Can you work these out from the model? Positions are in its coordinate system, mm. Give positions to 0.01 mm unless a question says otherwise; leave off trailing zeros. Order: outer loops, then holes, each group sorted by start corner. A loop starts at its lowest first (then second) coordinate and runs counter-clockwise, first axis right, second up. Notation, with made-up numbers: (77.25, 72) - (86.25, 72) arc R26 ccw to (86.25, 110) - close; hole circle Ø4 at (35.25, 82). An arc over 180 degrees is marked (long way). Write each question's results on one line, items separated by ' | '. Start each with the question number.
Autodesk Inventor part; units mm, degrees
ref_plane "YZ Plane" through (0, 0, 0) normal (1, 0, 0) x (0, 1, 0)
ref_plane "XZ Plane" through (0, 0, 0) normal (0, 1, 0) x (-1, 0, 0)
ref_plane "XY Plane" through (0, 0, 0) normal (0, 0, 1) x (1, 0, 0)
sketch "Skizze_1" plane through (0, 0, 0) normal (0, 0, 1) x (1, 0, 0)
  line L0 (-17.5, 0) -> (-17.5, -1)
  line L1 (-17.5, -1) -> (-13.5, -1)
  line L2 (-13.5, -1) -> (-13.5, -7.5)
  line L3 (-13.5, -7.5) -> (13.5, -7.5)
  line L4 (13.5, -7.5) -> (13.5, -1)
  line L5 (13.5, -1) -> (17.5, -1)
  line L6 (17.5, -1) -> (17.5, 0)
  line L7 (17.5, 0) -> (12.5, 0)
  line L8 (12.5, 0) -> (12.5, -6.5)
  line L9 (12.5, -6.5) -> (-12.5, -6.5)
  line L10 (-12.5, -6.5) -> (-12.5, 0)
  line L11 (-12.5, 0) -> (-17.5, 0)
extrude "Extrusion1" add sketch "Skizze_1" along normal blind 350
sketch "sketch_roundrect_1" plane through (0, 0, 0) normal (0, 1, 0) x (-1, 0, 0)
  arc A0 (2.6, 9.9) -> (-2.6, 9.9) centre (0, 9.9) ccw
  line L0 (-2.6, 9.9) -> (-2.6, -9.9)
  arc A1 (-2.6, -9.9) -> (2.6, -9.9) centre (0, -9.9) ccw
  line L1 (2.6, -9.9) -> (2.6, 9.9)
extrude "Extrusion2" cut sketch "sketch_roundrect_1" against normal blind 50
sketch "sketch_roundrect_2" plane through (0, 0, 0) normal (0, 1, 0) x (-1, 0, 0)
  arc A0 (2.6, 45.9) -> (-2.6, 45.9) centre (0, 45.9) ccw
  line L0 (-2.6, 45.9) -> (-2.6, 26.1)
  arc A1 (-2.6, 26.1) -> (2.6, 26.1) centre (0, 26.1) ccw
  line L1 (2.6, 26.1) -> (2.6, 45.9)
extrude "Extrusion3" cut sketch "sketch_roundrect_2" against normal blind 50
sketch "sketch_roundrect_3" plane through (0, 0, 0) normal (0, 1, 0) x (-1, 0, 0)
  arc A0 (2.6, 81.9) -> (-2.6, 81.9) centre (0, 81.9) ccw
  line L0 (-2.6, 81.9) -> (-2.6, 62.1)
  arc A1 (-2.6, 62.1) -> (2.6, 62.1) centre (0, 62.1) ccw
  line L1 (2.6, 62.1) -> (2.6, 81.9)
extrude "Extrusion4" cut sketch "sketch_roundrect_3" against normal blind 50
sketch "sketch_roundrect_4" plane through (0, 0, 0) normal (0, 1, 0) x (-1, 0, 0)
  arc A0 (2.6, 117.9) -> (-2.6, 117.9) centre (0, 117.9) ccw
  line L0 (-2.6, 117.9) -> (-2.6, 98.1)
  arc A1 (-2.6, 98.1) -> (2.6, 98.1) centre (0, 98.1) ccw
  line L1 (2.6, 98.1) -> (2.6, 117.9)
extrude "Extrusion5" cut sketch "sketch_roundrect_4" against normal blind 50
sketch "sketch_roundrect_5" plane through (0, 0, 0) normal (0, 1, 0) x (-1, 0, 0)
  arc A0 (2.6, 153.9) -> (-2.6, 153.9) centre (0, 153.9) ccw
  line L0 (-2.6, 153.9) -> (-2.6, 134.1)
  arc A1 (-2.6, 134.1) -> (2.6, 134.1) centre (0, 134.1) ccw
  line L1 (2.6, 134.1) -> (2.6, 153.9)
extrude "Extrusion6" cut sketch "sketch_roundrect_5" against normal blind 50
sketch "sketch_roundrect_6" plane through (0, 0, 0) normal (0, 1, 0) x (-1, 0, 0)
  arc A0 (2.6, 189.9) -> (-2.6, 189.9) centre (0, 189.9) ccw
  line L0 (-2.6, 189.9) -> (-2.6, 170.1)
  arc A1 (-2.6, 170.1) -> (2.6, 170.1) centre (0, 170.1) ccw
  line L1 (2.6, 170.1) -> (2.6, 189.9)
extrude "Extrusion7" cut sketch "sketch_roundrect_6" against normal blind 50
sketch "sketch_roundrect_7" plane through (0, 0, 0) normal (0, 1, 0) x (-1, 0, 0)
  arc A0 (2.6, 225.9) -> (-2.6, 225.9) centre (0, 225.9) ccw
  line L0 (-2.6, 225.9) -> (-2.6, 206.1)
  arc A1 (-2.6, 206.1) -> (2.6, 206.1) centre (0, 206.1) ccw
  line L1 (2.6, 206.1) -> (2.6, 225.9)
extrude "Extrusion8" cut sketch "sketch_roundrect_7" against normal blind 50
sketch "sketch_roundrect_8" plane through (0, 0, 0) normal (0, 1, 0) x (-1, 0, 0)
  arc A0 (2.6, 261.9) -> (-2.6, 261.9) centre (0, 261.9) ccw
  line L0 (-2.6, 261.9) -> (-2.6, 242.1)
  arc A1 (-2.6, 242.1) -> (2.6, 242.1) centre (0, 242.1) ccw
  line L1 (2.6, 242.1) -> (2.6, 261.9)
extrude "Extrusion9" cut sketch "sketch_roundrect_8" against normal blind 50
sketch "sketch_roundrect_9" plane through (0, 0, 0) normal (0, 1, 0) x (-1, 0, 0)
  arc A0 (2.6, 297.9) -> (-2.6, 297.9) centre (0, 297.9) ccw
  line L0 (-2.6, 297.9) -> (-2.6, 278.1)
  arc A1 (-2.6, 278.1) -> (2.6, 278.1) centre (0, 278.1) ccw
  line L1 (2.6, 278.1) -> (2.6, 297.9)
extrude "Extrusion10" cut sketch "sketch_roundrect_9" against normal blind 50
sketch "sketch_roundrect_10" plane through (0, 0, 0) normal (0, 1, 0) x (-1, 0, 0)
  arc A0 (2.6, 333.9) -> (-2.6, 333.9) centre (0, 333.9) ccw
  line L0 (-2.6, 333.9) -> (-2.6, 314.1)
  arc A1 (-2.6, 314.1) -> (2.6, 314.1) centre (0, 314.1) ccw
  line L1 (2.6, 314.1) -> (2.6, 333.9)
extrude "Extrusion11" cut sketch "sketch_roundrect_10" against normal blind 50
sketch "sketch_roundrect_11" plane through (0, 0, 0) normal (0, 1, 0) x (-1, 0, 0)
  arc A0 (2.6, 369.9) -> (-2.6, 369.9) centre (0, 369.9) ccw
  line L0 (-2.6, 369.9) -> (-2.6, 350.1)
  arc A1 (-2.6, 350.1) -> (2.6, 350.1) centre (0, 350.1) ccw
  line L1 (2.6, 350.1) -> (2.6, 369.9)
extrude "Extrusion12" cut sketch "sketch_roundrect_11" against normal blind 50
properties part number "WAGO_210-112350"
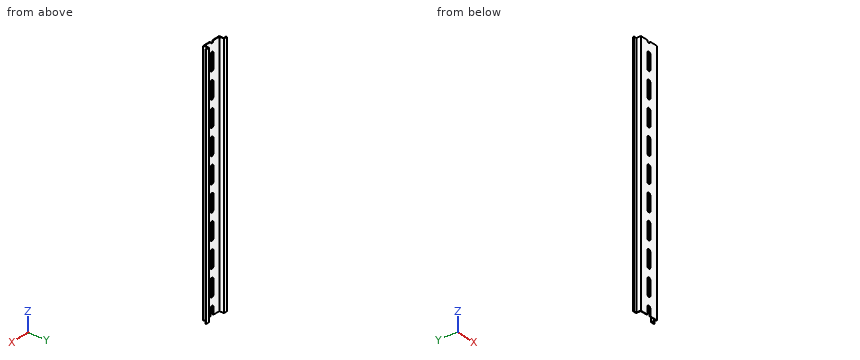
Q1. If we section it at C-C (x = -7): Please give me the cut outline in (y, z).
Q2. Will these pins go through, and if not, where does the flat tip stop? P1, Ø1.1, axis at y = -7, z = 104.5, coming from the +X side; P2, Ø4, axis at x = -5, z = 126.5, coming from the +Y side; P3, Ø0.8, axis at y = -7, z = 216, coming from the -X side.
Q3. If we section it at B-B (z = 254): Please give me the cut outline in (x, y), plus the area to 3 significant figures.
Q4. If I drill on probe 1 along X at (y, z) = (-4.75, 259.5); probe 2 along X at (y, z) = (-0.75, 198); probe 3 along Y at (x, z) = (-16, 181.5), over which ranges is the centre line in solid material (lowest first)? Write a range as from..to.
Q5. If we section it at A-A (y = -4.75): Please give me the cut outline in (x, z).
Findings below:
1) outline: (-7.5, 0) - (-6.5, 0) - (-6.5, 350) - (-7.5, 350) - close
2) P1: stops at x = 13.5 | P2: stops at y = -6.5 | P3: stops at x = -13.5
3) outline: (-17.5, -1) - (-13.5, -1) - (-13.5, -7.5) - (-2.6, -7.5) - (-2.6, -6.5) - (-12.5, -6.5) - (-12.5, 0) - (-17.5, 0) - close; (2.6, -7.5) - (13.5, -7.5) - (13.5, -1) - (17.5, -1) - (17.5, 0) - (12.5, 0) - (12.5, -6.5) - (2.6, -6.5) - close | area: 42.8 mm2
4) probe 1: x = -13.5..-12.5, 12.5..13.5 | probe 2: x = -17.5..-12.5, 12.5..17.5 | probe 3: y = -1..0
5) outline: (-13.5, 0) - (-12.5, 0) - (-12.5, 350) - (-13.5, 350) - close; (12.5, 0) - (13.5, 0) - (13.5, 350) - (12.5, 350) - close
